Print and shaded views of the part. All mm, measured from the part's lowest x, y and z. A direction names the side the tool comes from. Round coordinates to 2 decimals unless told otherwise and drop trailing zeros. Loops run counter-clockwise (first coordinate to the right, second up) from the corner with the lowest first, then second, coordinate; pieces in that order, holes last. Notation, with made-up numbers: (-37.75, 42) -> (-20.75, 42) arc R8 ccw to (-20.75, 55) -> close; hole circle Ø5 at (-19.5, 88.25). An arc over 180 degrees is marked (long way). Answer as CSV lines item,"result".
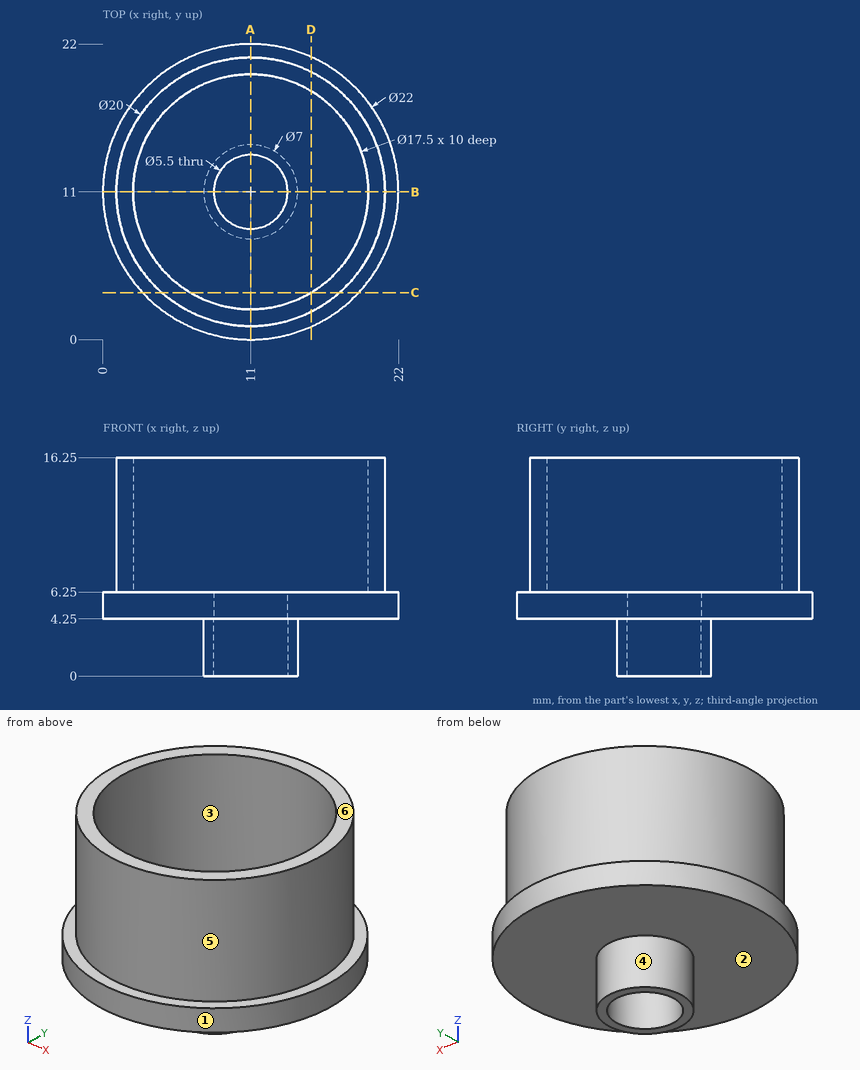
Q1. Tool access for the marked faces 4, 5 and 6: list every direction of +Z, -Z, +X, -X, +Y, -Y with a clear straight run to the whole face (end or side of a thin tool).
Results:
face 4,"-Z"
face 5,"+Z"
face 6,"+Z, +X, -X, +Y, -Y"
Q2. Slice it at D-D, the plane x = 15.5. Give the cut face in (y, z).
Results:
outline,"(0.96, 4.25) -> (21.04, 4.25) -> (21.04, 6.25) -> (19.93, 6.25) -> (19.93, 16.25) -> (18.5, 16.25) -> (18.5, 6.25) -> (3.5, 6.25) -> (3.5, 16.25) -> (2.07, 16.25) -> (2.07, 6.25) -> (0.96, 6.25) -> close"
Q3. Slice it at C-C, the plane y = 3.5. Give the cut face in (x, z).
Results:
outline,"(2.95, 4.25) -> (19.05, 4.25) -> (19.05, 6.25) -> (17.61, 6.25) -> (17.61, 16.25) -> (15.51, 16.25) -> (15.51, 6.25) -> (6.49, 6.25) -> (6.49, 16.25) -> (4.39, 16.25) -> (4.39, 6.25) -> (2.95, 6.25) -> close"
Q4. Drop flat-ended pins along their axis: pin 1 Ø9 at (x, y) = (12, 12) entering from +Z; pin 2 Ø6 at (y, z) = (19, 6.5) entering from +X; pin 3 Ø1.5 at (x, z) = (6, 3) entering from +Y; pin 4 Ø2 at (y, z) = (4.5, 8.5) entering from -X. Give the stop position or say it passes through.
Results:
pin 1,"z = 6.25"
pin 2,"x = 20.79"
pin 3,"through"
pin 4,"x = 2.65"
Q5. Two-plate mould, pull along X, no slides. Class the marked faces 1, 2 and 3: pulls with the +X half, pulls with the -X half, needs draft (parallel to the pull), parting line crosses it, or undercut.
Results:
face 1,"parting line crosses it"
face 2,"needs draft"
face 3,"undercut"
Q6. Probe L1, parallel to X at y = 11, z = 13.5; L2, parallel to Y at x = 11, z = 3.4; L3, parallel to Y at x = 11, z = 4.85. List the from-to ranges inside material, lowest first. Write a range as [from, to].
Results:
L1,"[1, 2.25], [19.75, 21]"
L2,"[7.5, 8.25], [13.75, 14.5]"
L3,"[0, 8.25], [13.75, 22]"
Q7. Slice it at A-A, the plane x = 11. Give the cut face in (y, z), and give its area (3 significant figures).
Results:
outline,"(0, 4.25) -> (7.5, 4.25) -> (7.5, 0) -> (8.25, 0) -> (8.25, 6.25) -> (2.25, 6.25) -> (2.25, 16.25) -> (1, 16.25) -> (1, 6.25) -> (0, 6.25) -> close; (13.75, 0) -> (14.5, 0) -> (14.5, 4.25) -> (22, 4.25) -> (22, 6.25) -> (21, 6.25) -> (21, 16.25) -> (19.75, 16.25) -> (19.75, 6.25) -> (13.75, 6.25) -> close"
area,"64.4 mm2"
